Part model, mm, in its own coordinate system. Round coordinates to 2 decimals unless told otherwise and drop trailing zeros. Loops run counter-clockwise (first coordinate to the right, second up) from the corner with the lowest first, then second, coordinate; pieces in that order, holes last.
1) Band-saw the part on C-C, the plane y = 2. Write the cut outline in (x, z).
2) Band-saw the part on B-B, the plane y = 23. Write the cut outline in (x, z).
3) Probe line 1 (Z direction, x = 15, y = 21.5); line 2 (Z direction, x = 8, y = 15); line 3 (Y direction, x = -17.5, z = 25.5). List the from-to ranges inside material, lowest first.
4) Band-saw the part on A-A, the plane x = 26. Write the cut outline in (y, z).
5) Drop flat-ended pins along their axis: P1, Ø4, axis at x = 30, y = -8.5, coming from the +Z side; P2, Ø2, axis at x = -2, y = 5, coming from the -Z side; P3, Ø6, axis at x = 24, y = 15, coming from the +Z side. Give the stop position or say it passes through.
from build123d import *

# Parameters (mm, degrees)
SKETCH2_W           = 80
SKETCH2_H           = 60
BOSS_EXTRUDE1_DEPTH = 550
CUT_EXTRUDE3_DEPTH  = 80


with BuildPart() as part:
    # Sketch2 → Boss-Extrude1 (new body)
    with BuildSketch(Plane.XY):
        Rectangle(SKETCH2_W, SKETCH2_H)
    extrude(amount=BOSS_EXTRUDE1_DEPTH)

    # Sketch4 → Cut-Extrude3 (cut)
    with BuildSketch(Plane(origin=(40, 0, 0), x_dir=(0, 0, -1), z_dir=(1, 0, 0))):
        Polygon((-550, 30), (-550, -8.699429877), (-500, 30), align=None)
        Polygon((-50, 30), (0, -8.699429877), (0, 30), align=None)
    extrude(amount=-CUT_EXTRUDE3_DEPTH, mode=Mode.SUBTRACT)


solid = part.part
Reported:
1. outline: (-40, 13.82) - (40, 13.82) - (40, 536.18) - (-40, 536.18) - close
2. outline: (-40, 40.96) - (40, 40.96) - (40, 509.04) - (-40, 509.04) - close
3. line 1: z = 39.02 to 510.98
3. line 2: z = 30.62 to 519.38
3. line 3: y = -30 to 11.04
4. outline: (-30, 0) - (-8.7, 0) - (30, 50) - (30, 500) - (-8.7, 550) - (-30, 550) - close
5. P1: stops at z = 550
5. P2: stops at z = 16.41
5. P3: stops at z = 523.26
